```python
from build123d import *

# Parameters (mm, degrees)
F0_R     = 12.7
F0_R_2   = 1.68372
F0_R_3   = 6.35
F1_DEPTH = 25.4
F0_R_4   = 4.0005
F2_DEPTH = 7.62
F3_DEPTH = 7.62


with BuildPart() as f1:
    # F0 (on Top) → F1 (new body)
    with BuildSketch(Plane.XY):
        Circle(F0_R)
        with Locations((-6.423387, -7.064583)):
            Circle(F0_R_2, mode=Mode.SUBTRACT)
        with Locations((6.204293, -7.064583)):
            Circle(F0_R_2, mode=Mode.SUBTRACT)
        Circle(F0_R_3, mode=Mode.SUBTRACT)
        with Locations((-6.423387, 7.338002)):
            Circle(F0_R_2, mode=Mode.SUBTRACT)
        with Locations((7.240649, 7.338002)):
            Circle(F0_R_2, mode=Mode.SUBTRACT)
    extrude(amount=F1_DEPTH)

    # F0 (on Top) → F2 (join)
    with BuildSketch(Plane.XY):
        Circle(F0_R_3)
        Circle(F0_R_4, mode=Mode.SUBTRACT)
    extrude(amount=F2_DEPTH)

    # F0 (on Top) → F3 (join)
    with BuildSketch(Plane.XY):
        Circle(F0_R_4)
    extrude(amount=F3_DEPTH)


solid = f1.part
```
The listing builds one solid part. Answer for the finished solid, in the listing's coordinates (mm). A direction names the side the tool comes from. Give positions to 0.01 mm unless a question says otherwise; leave off trailing zeros. Order: outer loops, then holes, each group sorted by start corner. A loop starts at its lowest first (then second) coordinate and runs counter-clockwise, first axis right, second up. Notation, with made-up numbers: (67, 24.25) -> (124, 24.25) arc R16 ccw to (124, 41.25) -> close; hole circle Ø6 at (-32.5, -24). An arc over 180 degrees is marked (long way). One line per item, written item: value.
1) Determine the mould class of faces 1 (the cylindrical face through (8.8, 6.7, 12.5)), 2 (the cylindrical face through (-2.75, -12.4, 12.52)), 3 (the flat face through (-6, -3, 25.4)) for opening direction X: pulls with the +X half, pulls with the -X half, needs draft (parallel to the pull), parting line crosses it, or undercut.
Reported:
face 1: undercut
face 2: parting line crosses it
face 3: needs draft
2) Find section A-A, the plane x = 0. Determine the outline of the cut face in (y, z).
Reported:
outline: (-12.7, 0) -> (12.7, 0) -> (12.7, 25.4) -> (6.35, 25.4) -> (6.35, 7.62) -> (-6.35, 7.62) -> (-6.35, 25.4) -> (-12.7, 25.4) -> close
3) Find section B-B, the plane y = -7.5. Determine the outline of the cut face in (x, z).
Reported:
outline: (-10.25, 0) -> (-8.05, 0) -> (-8.05, 25.4) -> (-10.25, 25.4) -> close; (-4.8, 0) -> (4.58, 0) -> (4.58, 25.4) -> (-4.8, 25.4) -> close; (7.83, 0) -> (10.25, 0) -> (10.25, 25.4) -> (7.83, 25.4) -> close
4) Find section D-D, the plane z = 11. Determine the outline of the cut face in (x, y), plus the area to 3 significant figures.
Reported:
outline: circle Ø25.4 at (0, 0); hole circle Ø3.37 at (-6.42, -7.06); hole circle Ø3.37 at (-6.42, 7.34); hole circle Ø12.7 at (0, 0); hole circle Ø3.37 at (6.2, -7.06); hole circle Ø3.37 at (7.24, 7.34)
area: 344 mm^2
5) Find the intervals of material crossed by line 1 (X direction, y = 8, z = 5.5); line 2 (Y direction, x = -5, z = 19.75); line 3 (X direction, y = 0.25, z = 13.5), in increasing order.
Reported:
line 1: x = -9.86 to -7.97, -4.88 to 5.69, 8.79 to 9.86
line 2: y = -11.67 to -7.96, -6.17 to -3.91, 3.91 to 6.44, 8.24 to 11.67
line 3: x = -12.7 to -6.35, 6.35 to 12.7
6) Flat-ended cylindrical pins translate along their axes: P1, Ø14, axis at x = 0.5, y = 0.5, coming from the +Z side; P2, Ø1, axis at x = 2, y = -0.5, coming from the +Z side; P3, Ø6, axis at y = -10, z = 7, coming from the +X side; P4, Ø5, axis at y = 6.5, z = 5, coming from the -X side. Find the tip coordinate at first contact, or state that the pin passes through.
Reported:
P1: stops at z = 25.4
P2: stops at z = 7.62
P3: stops at x = 10.6
P4: stops at x = -12.05
7) A tool of negligible diameter and unlimited length cuts with its end or side. For faces 4 (the cylindrical face through (-6.788, 5.694, 12.522)), 5 (the cylindrical face through (-1.38, -6.2, 16.39)), from which of +Z, -Z, +X, -X, +Y, -Y can it reach the whole face along a straight path? Write none if from no direction.
Reported:
face 4: +Z, -Z
face 5: +Z
